Read the model definition and answer for the solid it produces. Units are mm, in the model's axes. Round coordinates to 2 decimals unless told otherwise and drop trailing zeros. Loops run counter-clockwise (first coordinate to the right, second up) from the corner with the lowest first, then second, coordinate; pieces in that order, holes last. Notation, with made-up numbers: (5.25, 10) - (10.25, 10) arc R20 ccw to (10.25, 20) - close; hole circle Ø1 at (46, -23.75). An arc over 180 degrees is marked (long way). Use one line per item in the form item = value. Start each with the question number.
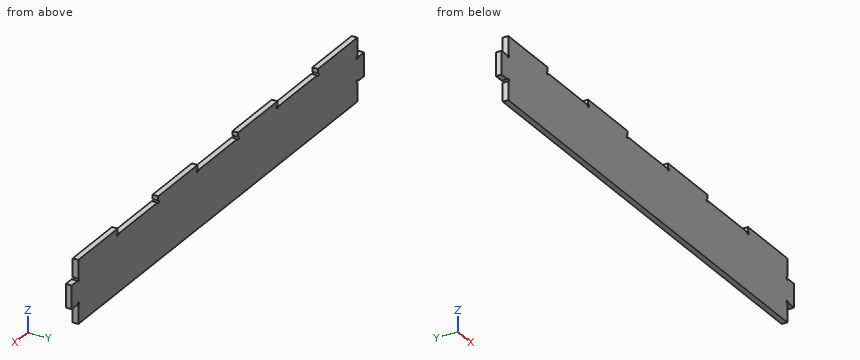
Autodesk Inventor part; units mm, degrees
ref_plane "YZ Plane" through (0, 0, 0) normal (1, 0, 0) x (0, 1, 0)
ref_plane "XZ Plane" through (0, 0, 0) normal (0, 1, 0) x (-1, 0, 0)
ref_plane "XY Plane" through (0, 0, 0) normal (0, 0, 1) x (1, 0, 0)
sketch "Sketch1" plane through (0, 0, 0) normal (0, 1, 0) x (-1, 0, 0)
  line L0 (173, 22.25) -> (-173, 22.25)
  line L1 (-173, 22.25) -> (-173, -22.25)
  line L2 (-173, -22.25) -> (173, -22.25)
  line L3 (173, -22.25) -> (173, 22.25)
  point P0 (0, 0)
  point P1 (0, -22.25)
  point P2 (173, 0)
  dimension "d0" = 44.5
  dimension "d1" = 346
extrude "Extrusion1" add sketch "Sketch1" along normal blind 4
sketch "Esboço2" plane through (0, 4, 0) normal (0, 1, 0) x (1, 0, 0)
  line L0 (-173, -22.25) -> (173, -22.25)
  line L1 (-118.5, -22.25) -> (-70.5, -22.25)
  line L2 (-70.5, -22.25) -> (-70.5, -18.25)
  line L3 (-70.5, -18.25) -> (-118.5, -18.25)
  line L4 (-118.5, -18.25) -> (-118.5, -22.25)
  line L5 (-173, 22.25) -> (-173, -22.25)
  line L6 (-24, -22.25) -> (24, -22.25)
  line L7 (24, -22.25) -> (24, -18.25)
  line L8 (24, -18.25) -> (-24, -18.25)
  line L9 (-24, -18.25) -> (-24, -22.25)
  line L10 (70.5, -22.25) -> (118.5, -22.25)
  line L11 (118.5, -22.25) -> (118.5, -18.25)
  line L12 (118.5, -18.25) -> (70.5, -18.25)
  line L13 (70.5, -18.25) -> (70.5, -22.25)
  circle A0 centre (-118.5, -18.25) radius 1
  circle A1 centre (-70.5, -18.25) radius 1
  circle A2 centre (-24, -18.25) radius 1
  circle A3 centre (24, -18.25) radius 1
  circle A4 centre (70.5, -18.25) radius 1
  circle A5 centre (118.5, -18.25) radius 1
  point P0 (0, 0)
  dimension "d4" = 48
  dimension "d5" = 4
  dimension "d6" = 54.5
  dimension "d7" = 48
  dimension "d8" = 48
  dimension "d9" = 46.5
  dimension "d10" = 46.5
  dimension "d11" = 2
  dimension "d12" = 2
  dimension "d13" = 2
  dimension "d14" = 2
  dimension "d15" = 2
  dimension "d16" = 2
extrude "Extrusão2" cut sketch "Esboço2" against normal blind 10
sketch "Esboço3" plane through (0, 4, 0) normal (0, 1, 0) x (1, 0, 0)
  line L0 (-173, 22.25) -> (-173, -22.25)
  line L1 (-173, 22.25) -> (-165, 22.25)
  line L2 (-165, 22.25) -> (-165, 8.25)
  line L3 (-165, 8.25) -> (-173, 8.25)
  line L4 (-173, 8.25) -> (-173, 22.25)
  line L5 (-173, -22.25) -> (-165, -22.25)
  line L6 (-165, -22.25) -> (-165, -8.25)
  line L7 (-165, -8.25) -> (-173, -8.25)
  line L8 (-173, -8.25) -> (-173, -22.25)
  circle A0 centre (-165, 8.25) radius 1
  circle A1 centre (-165, -8.25) radius 1
  point P0 (0, 0)
  dimension "d19" = 8
  dimension "d20" = 14
  dimension "d21" = 14
  dimension "d22" = 16.5
  dimension "d23" = 2
  dimension "d24" = 2
extrude "Extrusão3" cut sketch "Esboço3" against normal blind 10
mirror "Espelhamento1" about plane through (0, 0, 0) normal (1, 0, 0) of "Extrusão3"
properties part number "fechamento inferior"
1) Flat-ended cylindrical pins translate along their axes: pin 1 (8 mm diameter, centred on x = -120.5, z = 6, fed in from -Y); pin 2 (1.5 mm diameter, centred on y = 2, z = 21, fed in from -X); pin 3 (1.2 mm diameter, centred on y = 2.5, z = -17.5, fed in from +X); pin 4 (1.2 mm diameter, centred on x = 165, z = -8.25, fed in from +Y). Find the tip coordinate at first contact, or state that the pin passes through.
2) A cutting plane is placed at B-B on x = 84.5. Write down the section's boundary in (y, z).
3) Straight lines are drawn through the part: line 1 (X direction, y = 3.3, z = 20.5); line 2 (X direction, y = 2.5, z = -8); line 3 (Z direction, x = -0.5, y = 1.8). For each, find the intervals that lie inside material, in ascending order. Write a range as from..to.
Checks:
q1.pin_1 = 0
q1.pin_2 = -165
q1.pin_3 = 165
q1.pin_4 = through
q2.outline = (0, -22.25) - (4, -22.25) - (4, 18.25) - (0, 18.25) - close
q3.line_1 = -165..-118.5, -70.5..-24, 24..70.5, 118.5..165
q3.line_2 = -173..-165.97, -164.03..164.03, 165.97..173
q3.line_3 = -22.25..18.25
